from build123d import *

# Parameters (mm, degrees)
SKETCH1_W           = 25.4
SKETCH1_H           = 25.4
BOSS_EXTRUDE1_DEPTH = 3.175
CUT_EXTRUDE1_DEPTH  = 4.175


with BuildPart() as part:
    # Sketch1 → Boss-Extrude1 (new body)
    with BuildSketch(Plane.XY):
        Polygon((0, 0), (19.05, 0), (19.05, -6.35), (57.15, -6.35), (57.15, 0), (76.2, 0), (76.2, 3.175), (73.66, 3.175), (73.66, 28.575), (76.2, 28.575), (76.2, 31.75), (57.15, 31.75), (57.15, 34.925), (19.05, 34.925), (19.05, 31.75), (0, 31.75), (0, 28.575), (2.54, 28.575), (2.54, 3.175), (0, 3.175), align=None)
        with Locations((38.1, 15.875)):
            Rectangle(SKETCH1_W, SKETCH1_H, mode=Mode.SUBTRACT)
    extrude(amount=BOSS_EXTRUDE1_DEPTH)

    # Sketch2 → Cut-Extrude1 (cut, through all)
    with BuildSketch(Plane.XY.offset(3.175)):
        Polygon((13.03, 0), (9.83, 0), (9.83, 6.5), (8.63, 6.5), (8.63, 8.5), (9.83, 8.5), (9.83, 10), (13.03, 10), (13.03, 8.5), (14.23, 8.5), (14.23, 6.5), (13.03, 6.5), align=None)
        Polygon((66.37, 8.5), (66.37, 10), (63.17, 10), (63.17, 8.5), (61.97, 8.5), (61.97, 6.5), (63.17, 6.5), (63.17, 0), (66.37, 0), (66.37, 6.5), (67.57, 6.5), (67.57, 8.5), align=None)
    extrude(amount=-CUT_EXTRUDE1_DEPTH, mode=Mode.SUBTRACT)


solid = part.part
For this review, take the finished solid that the model builds, in its own axes (mm). A direction names the side the tool comes from. Round coordinates to 2 decimals unless told otherwise and drop trailing zeros. Loops run counter-clockwise (first coordinate to the right, second up) from the corner with the lowest first, then second, coordinate; pieces in that order, holes last. Notation, with made-up numbers: (14.5, 55.25) - (34.5, 55.25) arc R18 cw to (34.5, 72.25) - close; hole circle Ø3 at (26, -29). An arc over 180 degrees is marked (long way). One line per item, written item: value. Start each with the question number.
Item 1: Take a section at D-D (x = 18). Give the boundary of the cut face in (y, z) (3 decimals), plus the area to 3 significant figures.
Item 2: Take a section at A-A (y = 5). Give the boundary of the cut face in (x, z) (3 decimals).
Item 3: Take a section at C-C (y = 18.5). Give the boundary of the cut face in (x, z) (3 decimals), plus the area to 3 significant figures.
Item 4: For L1, parallel to Y at x = 41, z = 2.65 (3 decimals); L2, parallel to X at y = 26, z = 1.9; L3, parallel to X at y = 2, z = 2.55, list the stretches that pass through material, from the lowest coordinate up.
Item 5: Take a section at B-B (x = 27.5). Give the boundary of the cut face in (y, z) (3 decimals), plus the area to 3 significant figures.
Item 6: The part is to be moulded in two halves that separate along X. For faces 5 (the flat face through (38, 3.175, 2)), 6 (the flat face through (2.54, 16, 2)), 7 (the flat face through (76.2, 30, 2)), 8 (the flat face through (38, 34.925, 2)), say which applies: +X half, -X half, draft (parallel to the pull), parting line (faces both ways), or undercut.
Item 7: For faces 1 (the flat face through (71, 0, 2)), 2 (the flat face through (63.17, 9, 2)), 3 (the flat face through (5, 0, 2)), 4 (the flat face through (75, 3.175, 2)), list the 3-axis set-ups (+Z, -Z, +X, -X, +Y, -Y) from which the entire face can be reached by the end or side of a thin tool; tool diameter is ignored.
Item 8: Clearance check with flat-ended pins moving along their axes: pin 1 Ø1.6 at (x, z) = (3.5, 1) entering from -Y; pin 2 Ø1 at (x, z) = (67, 1) entering from +Y; pin 3 Ø1.6 at (y, z) = (7.5, 1) entering from -X. State where each tip first meets the part, or that it passes through.
Answer below:
1. outline: (0, 0) - (31.75, 0) - (31.75, 3.175) - (0, 3.175) - close
1. area: 101 mm2
2. outline: (2.54, 0) - (9.83, 0) - (9.83, 3.175) - (2.54, 3.175) - close; (13.03, 0) - (25.4, 0) - (25.4, 3.175) - (13.03, 3.175) - close; (50.8, 0) - (63.17, 0) - (63.17, 3.175) - (50.8, 3.175) - close; (66.37, 0) - (73.66, 0) - (73.66, 3.175) - (66.37, 3.175) - close
3. outline: (2.54, 0) - (25.4, 0) - (25.4, 3.175) - (2.54, 3.175) - close; (50.8, 0) - (73.66, 0) - (73.66, 3.175) - (50.8, 3.175) - close
3. area: 145 mm2
4. L1: y = -6.35 to 3.175, 28.575 to 34.925
4. L2: x = 2.54 to 25.4, 50.8 to 73.66
4. L3: x = 0 to 9.83, 13.03 to 63.17, 66.37 to 76.2
5. outline: (-6.35, 0) - (3.175, 0) - (3.175, 3.175) - (-6.35, 3.175) - close; (28.575, 0) - (34.925, 0) - (34.925, 3.175) - (28.575, 3.175) - close
5. area: 50.4 mm2
6. face 5: undercut
6. face 6: -X half
6. face 7: +X half
6. face 8: draft
7. face 1: +Z, -Z, +X, -Y
7. face 2: +Z, -Z, -Y
7. face 3: +Z, -Z, -X, -Y
7. face 4: +Z, -Z, +X
8. pin 1: stops at y = 0
8. pin 2: stops at y = 31.75
8. pin 3: stops at x = 2.54
